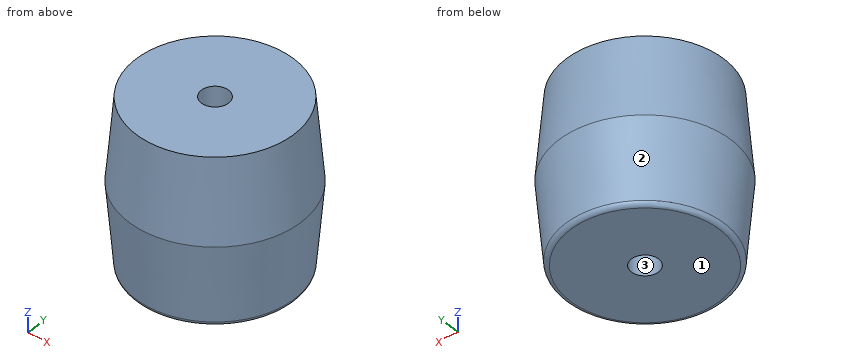
from build123d import *

# Parameters (mm, degrees)
SKETCH1_R                     = 9.5
BOSS_EXTRUDE1_DEPTH           = 9.1
BOSS_EXTRUDE1_TAPER           = 5
BOSS_EXTRUDE1_OTHER_WAY_DEPTH = 9.1
BOSS_EXTRUDE1_OTHER_WAY_TAPER = 5
FILLET1_R                     = 0.5
SKETCH2_R                     = 1.5
CUT_EXTRUDE1_DEPTH            = 18.5


with BuildPart() as part:
    # Sketch1 → Boss-Extrude1 (new body)
    with BuildSketch(Plane.XY):
        Circle(SKETCH1_R)
    extrude(amount=BOSS_EXTRUDE1_DEPTH, taper=BOSS_EXTRUDE1_TAPER)

    # Sketch1 → Boss-Extrude1 other way (add)
    with BuildSketch(Plane.XY):
        Circle(SKETCH1_R)
    extrude(amount=-BOSS_EXTRUDE1_OTHER_WAY_DEPTH, taper=BOSS_EXTRUDE1_OTHER_WAY_TAPER)

    # Fillet1
    fillet1_edges = [part.edges().sort_by_distance(p)[0] for p in [
        (-8.703853162, 0, -9.1),
    ]]
    fillet(fillet1_edges, radius=FILLET1_R)

    # Sketch2 → Cut-Extrude1 (cut)
    with BuildSketch(Plane.XY.offset(9.1)):
        Circle(SKETCH2_R)
    extrude(amount=-CUT_EXTRUDE1_DEPTH, mode=Mode.SUBTRACT)


solid = part.part
Verification items for the finished model (mm, model axes). Face numbers are marked on the shaded views. Coordinates: 2 decimals unless noted, no trailing zeros. Write each loop counter-clockwise with the first axis right and the second up, starting at its lowest first coordinate (ties: lowest second). Pieces come first, ordered by that corner, then holes. Notation, with made-up numbers: (42, -38.75) - (63, -38.75) arc R18 ccw to (63, -11.75) - close; hole circle Ø8 at (-30.5, 68). An arc over 180 degrees is marked (long way). Answer as a JSON object with one key per item and string values.
(1) Thickness scan on line 1 along Y through (x, z) = (0, 0); line 2 along Y through (x, z) = (0, 2.75); line 3 along Y through (x, z) = (-4.25, -2.5). Record the ranges inside material, lowest first.
Report:
{"line 1": "-9.5 to -1.5, 1.5 to 9.5", "line 2": "-9.26 to -1.5, 1.5 to 9.26", "line 3": "-8.25 to 8.25"}
(2) Cross-section at A-A on x = 0. Record the cut outline in (y, z).
Report:
{"outline": "(-9.5, 0) - (-8.74, -8.64) arc R0.5 ccw to (-8.25, -9.1) - (-1.5, -9.1) - (-1.5, 9.1) - (-8.7, 9.1) - close; (1.5, -9.1) - (8.25, -9.1) arc R0.5 ccw to (8.74, -8.64) - (9.5, 0) - (8.7, 9.1) - (1.5, 9.1) - close"}
(3) Gauge pin test, flat ends, axial feed: pin 1 Ø4 at (y, z) = (-6.5, -5) entering from -X; pin 2 Ø5 at (y, z) = (-3, 6) entering from -X; pin 3 Ø8 at (y, z) = (2.5, 4) entering from +X; pin 4 Ø1 at (x, y) = (7, -5) entering from -Z. Record the tip position at first contact, or that the pin passes through.
Report:
{"pin 1": "x = -7.88", "pin 2": "x = -9.05", "pin 3": "x = 9.44", "pin 4": "z = -9.1"}
(4) Cross-section at C-C on z = 3. Record the cut outline in (x, y).
Report:
{"outline": "circle Ø18.48 at (0, 0); hole circle Ø3 at (0, 0)"}
(5) Mould release check, pull along Y, two halves, no side actions. Record for the marked faces 1, 2 and 3: pulls with the +Y half, pulls with the -Y half, needs draft (parallel to the pull), parting line crosses it, or undercut.
Report:
{"face 1": "needs draft", "face 2": "parting line crosses it", "face 3": "undercut"}
(6) Cross-section at B-B on z = 1. Record the cut outline in (x, y), plus the area to 3 significant figures.
Report:
{"outline": "circle Ø18.83 at (0, 0); hole circle Ø3 at (0, 0)", "area": "271 mm^2"}
